Check sheet for the modelled part. Datum: model origin and axes. Units: mm. Face numbers are marked on the shaded views. Coordinates: 2 decimals unless noted, no trailing zeros. Order: outer loops, then holes, each group sorted by start corner. A loop starts at its lowest first (then second) coordinate and runs counter-clockwise, first axis right, second up.
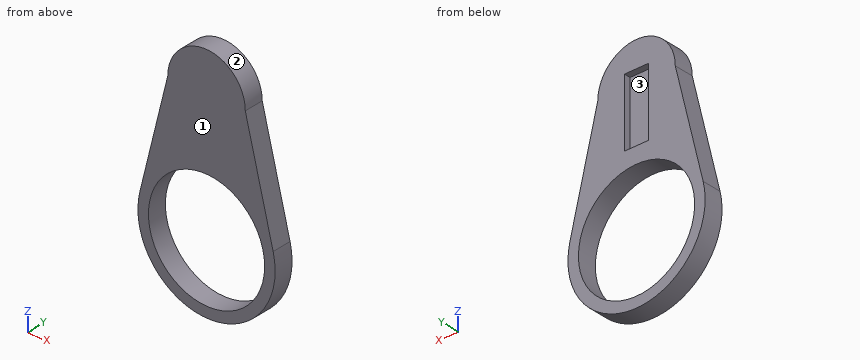
from build123d import *

# Parameters (mm, degrees)
SKETCH1_R           = 18
BOSS_EXTRUDE1_DEPTH = 6
SKETCH2_W           = 7.5
SKETCH2_H           = 21
CUT_EXTRUDE1_DEPTH  = 2


with BuildPart() as part:
    # Sketch1 → Boss-Extrude1 (new body)
    with BuildSketch(Plane(origin=(0, 0, 0), x_dir=(1, 0, 0), z_dir=(0, 1, 0))):
        with BuildLine():
            Line((-20.628820967, 34.89958379), (-12, 0))
            ThreePointArc((-12, 0), (0, -12), (12, 0))
            Line((12, 0), (20.628820967, 34.89958379))
            ThreePointArc((20.628820967, 34.89958379), (0, 61.25), (-20.628820967, 34.89958379))
        make_face()
        with Locations((0, 40)):
            Circle(SKETCH1_R, mode=Mode.SUBTRACT)
    extrude(amount=BOSS_EXTRUDE1_DEPTH)

    # Sketch2 → Cut-Extrude1 (cut)
    with BuildSketch(Plane(origin=(0, 6, 0), x_dir=(1, 0, 0), z_dir=(0, 1, 0))):
        with Locations((0, 6.5)):
            Rectangle(SKETCH2_W, SKETCH2_H)
    extrude(amount=-CUT_EXTRUDE1_DEPTH, mode=Mode.SUBTRACT)


solid = part.part
(1) Go/stop test with flat-tipped pins: P1, Ø1, axis at x = 0.5, y = 5, coming from the -Z side; P2, Ø1, axis at y = 1.5, z = -20, coming from the -X side; P3, Ø1, axis at y = 5.5, z = -5.5, coming from the +X side. Record where each tip stops, or that it passes through.
Filled in:
P1: stops at z = -61.25
P2: stops at x = -17.07
P3: stops at x = 13.48
(2) Cross-section at D-D (x = -6). Enter the section's corners in (y, z), and give its area (3 significant figures).
Filled in:
outline: (0, -60.39) - (6, -60.39) - (6, -56.97) - (0, -56.97) - close; (0, -23.03) - (6, -23.03) - (6, 10.39) - (0, 10.39) - close
area: 221 mm2
(3) Cross-section at C-C (y = 1.85). Enter the section's corners in (x, z).
Filled in:
outline: (-20.63, -34.9) arc R21.25 ccw (long way) to (20.63, -34.9) - (12, 0) arc R12 ccw to (-12, 0) - close; hole circle Ø36 at (0, -40)
(4) Thickness scan on probe 1 along Z at (x, y) = (0, 4.45); probe 2 along X at (y, z) = (2.8, -40); probe 3 along Z at (x, y) = (-0.5, 1.15). Record the ranges inside material, lowest first.
Filled in:
probe 1: z = -61.25 to -58, -22 to -17, 4 to 12
probe 2: x = -21.25 to -18, 18 to 21.25
probe 3: z = -61.24 to -57.99, -22.01 to 11.99
(5) Release check for a two-part mould opening along X. For the marked faces 1, 2 and 3 record: +X half, -X half, draft (parallel to the pull), parting line (faces both ways), or undercut.
Filled in:
face 1: draft
face 2: parting line
face 3: undercut
(6) Cross-section at B-B (x = 0). Enter the section's corners in (y, z).
Filled in:
outline: (0, -61.25) - (6, -61.25) - (6, -58) - (0, -58) - close; (0, -22) - (6, -22) - (6, -17) - (4, -17) - (4, 4) - (6, 4) - (6, 12) - (0, 12) - close
(7) Cross-section at A-A (z = -40). Enter the section's corners in (x, y).
Filled in:
outline: (-21.25, 0) - (-18, 0) - (-18, 6) - (-21.25, 6) - close; (18, 0) - (21.25, 0) - (21.25, 6) - (18, 6) - close
